Model file for the job. Use its own axes, mm. Face numbers are marked on the shaded views. Coordinates: 2 decimals unless noted, no trailing zeros. Order: outer loops, then holes, each group sorted by start corner. A loop starts at its lowest first (then second) coordinate and runs counter-clockwise, first axis right, second up. Notation, with made-up numbers: (25.5, 13) -> (39.5, 13) arc R21 ccw to (39.5, 42) -> close; hole circle Ø8 at (49, 0). An arc over 180 degrees is marked (long way). Write item = value, one per line. Start each with the question number.
Q1. Mould opens along Z. For the marked faces 1 and 2 say: +Z half, -Z half, draft (parallel to the pull), parting line (faces both ways), or undercut.
Q2. Cut at D-D, the plane x = -60. List the corners of the cut face in (y, z), plus the area to 3 significant figures.
Q3. Cut at C-C, the plane x = 51. List the corners of the cut face in (y, z).
Q4. Wall check: line 1 (Z direction, x = -15, y = -24.5); line 2 (Y direction, x = 84.5, z = -21.5); line 3 (Y direction, x = 42.5, z = -253). Give the ranges that are in metal, low to high. Write a range as from..to.
Q5. Cut at B-B, the plane y = -23.5. List the corners of the cut face in (x, z), plus the area to 3 significant figures.
Q6. Cut at A-A, the plane z = -196. List the corners of the cut face in (x, y).
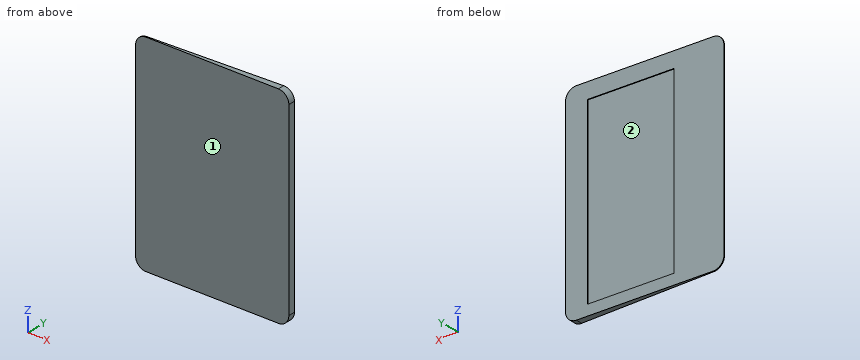
from build123d import *

# Parameters (mm, degrees)
F3_DEPTH = 300
F4_R     = 15
F5_R     = 15
F6_R     = 15
F7_R     = 15
F8_W     = 120.1740764081
F8_H     = 261.9301192462
F9_DEPTH = 1


with BuildPart() as f3:
    # F1 (on face) → F3 (new body)
    with BuildSketch(Plane.XY):
        Polygon((116.6105127335, -19.077671887), (-103.3894872665, -28.077671887), (-103.3894872665, -29.077671887), (116.6105127335, -29.077671887), align=None)
    extrude(amount=-F3_DEPTH)

    # F4
    f4_edges = [f3.edges().sort_by_distance(p)[0] for p in [
        (-103.389487, -28.577672, 0),
    ]]
    fillet(f4_edges, radius=F4_R)

    # F5
    f5_edges = [f3.edges().sort_by_distance(p)[0] for p in [
        (-103.389487, -28.577672, -300),
    ]]
    fillet(f5_edges, radius=F5_R)

    # F6
    f6_edges = [f3.edges().sort_by_distance(p)[0] for p in [
        (116.610513, -24.077672, -300),
    ]]
    fillet(f6_edges, radius=F6_R)

    # F7
    f7_edges = [f3.edges().sort_by_distance(p)[0] for p in [
        (116.610513, -24.077672, 0),
    ]]
    fillet(f7_edges, radius=F7_R)

    # F8 (on face) → F9 (cut)
    with BuildSketch(Plane(origin=(0.9739741727, -23.8082575553, 0), x_dir=(-0.999164272, -0.040874902, 0), z_dir=(-0.040874902, 0.999164272, 0))):
        with Locations((-25.0621605664, -153.7662539631)):
            Rectangle(F8_W, F8_H)
    extrude(amount=-F9_DEPTH, mode=Mode.SUBTRACT)


solid = f3.part
Here are the results:
q1.face_1 = draft
q1.face_2 = undercut
q2.outline = (-29.08, -300) -> (-26.3, -300) -> (-26.3, 0) -> (-29.08, 0) -> close
q2.area = 833 mm²
q3.outline = (-29.08, -300) -> (-21.76, -300) -> (-21.76, -284.73) -> (-22.76, -284.73) -> (-22.76, -22.8) -> (-21.76, -22.8) -> (-21.76, 0) -> (-29.08, 0) -> close
q4.line_1 = -300..-284.73, -22.8..0
q4.line_2 = -29.08..-20.39
q4.line_3 = -29.08..-23.11
q5.outline = (8.51, -300) -> (101.61, -300) arc R15 ccw to (116.61, -285) -> (116.61, -15) arc R15 ccw to (101.61, 0) -> (8.51, 0) -> (8.51, -22.8) -> (32.97, -22.8) -> (32.97, -284.73) -> (8.51, -284.73) -> close
q5.area = 25,900 mm²
q6.outline = (-103.39, -29.08) -> (116.61, -29.08) -> (116.61, -19.08) -> (86.05, -20.33) -> (86.09, -21.33) -> (-33.98, -26.24) -> (-34.02, -25.24) -> (-103.39, -28.08) -> close
